Check sheet for the modelled part. Datum: model origin and axes. Units: mm. Face numbers are marked on the shaded views. A direction names the side the tool comes from. Give positions to 0.01 mm unless a question says otherwise; leave off trailing zeros. Write each loop counter-clockwise with the first axis right and the second up, starting at its lowest first coordinate (ties: lowest second). Pieces come first, ordered by that corner, then holes. Notation, with made-up numbers: M 51.25,37 L 74.25,37 A24 ccw 74.25,63 Z; hole C 77,86 d4. An arc over 180 degrees is marked long. Use CSV: the item, a comma, the result in double quotes. Start each with the question number.
1. Scan lines: line 1 (Y direction, x = 0, z = 17.65); line 2 (Y direction, x = 0, z = -13.1); line 3 (Z direction, x = -8, y = -4.5). Record each from-to range of solid material in increasing order.
2. Depth check by flat-ended pin: P1, Ø1.6, axis at x = -8, y = 0.5, coming from the +Z side; P2, Ø1.5, axis at x = -2, z = -9, coming from the +Y side; P3, Ø5, axis at y = 6.5, z = 13.5, coming from the -X side. Enter the tip coordinate at first touch or a pass-through.
3. Access from +Z, -Z, +X, -X, +Y, -Y to the whole of each face (thin tool, end or side, straight path). Record for the marked faces 1 and 2.
4. Cross-section at C-C, the plane z = -0.5. Enter the section's corners in (x, y), and give its area (3 significant figures).
5. Cross-section at B-B, the plane y = 8.5. Enter the section's corners in (x, z).
6. Cross-section at A-A, the plane x = 0. Enter the section's corners in (y, z).
7. Cross-section at D-D, the plane x = -8. Enter the section's corners in (y, z), and give its area (3 significant figures).
from build123d import *

# Parameters (mm, degrees)
SKETCH1_R                = 10.25
BOSS_EXTRUDE1_DEPTH      = 19
BOSS_EXTRUDE1_DEPTH_BACK = 19
SKETCH2_R                = 4
BOSS_EXTRUDE2_DEPTH      = 1.9
SKETCH3_R                = 4
BOSS_EXTRUDE3_DEPTH      = 1
SKETCH4_R                = 1
CUT_EXTRUDE1_DEPTH       = 3.5
FILLET1_R                = 0.5
SKETCH7_R                = 10.25
CUT_EXTRUDE3_DEPTH       = 5.5
CUT_EXTRUDE3_DEPTH_BACK  = 3.5
SKETCH9_R                = 1.5
CUT_EXTRUDE5_DEPTH       = 5


with BuildPart() as part:
    # Sketch1 → Boss-Extrude1 (new body, two sides)
    with BuildSketch(Plane.XY) as boss_extrude1_sk:
        Circle(SKETCH1_R)
    extrude(amount=BOSS_EXTRUDE1_DEPTH)
    extrude(boss_extrude1_sk.sketch, amount=-BOSS_EXTRUDE1_DEPTH_BACK)

    # Sketch2 → Boss-Extrude2 (add)
    with BuildSketch(Plane.XY.offset(19)):
        Circle(SKETCH2_R)
    extrude(amount=BOSS_EXTRUDE2_DEPTH)

    # Sketch3 → Boss-Extrude3 (add)
    with BuildSketch(Plane(origin=(0, 0, -19), x_dir=(-1, 0, 0), z_dir=(0, 0, -1))):
        Circle(SKETCH3_R)
    extrude(amount=BOSS_EXTRUDE3_DEPTH)

    # Sketch4 → Cut-Extrude1 (cut)
    with BuildSketch(Plane.XY.offset(19)):
        with Locations((0, 8)):
            Circle(SKETCH4_R)
        with Locations((8, 0)):
            Circle(SKETCH4_R)
        with Locations((0, -8)):
            Circle(SKETCH4_R)
        with Locations((-8, 0)):
            Circle(SKETCH4_R)
    cut_extrude1 = extrude(amount=-CUT_EXTRUDE1_DEPTH, mode=Mode.SUBTRACT)

    # Fillet1
    fillet1_edges = [part.edges().sort_by_distance(p)[0] for p in [
        (-4, 0, 20.9),
    ]]
    fillet(fillet1_edges, radius=FILLET1_R)

    # Mirror1: Cut-Extrude1 across plane
    add(cut_extrude1.mirror(Plane(origin=(0, 0, 0), x_dir=(1, 0, 0), z_dir=(0, 0, -1))), mode=Mode.SUBTRACT)

    # Sketch7 → Cut-Extrude3 (cut, two sides)
    with BuildSketch(Plane(origin=(0, 0, -19), x_dir=(-1, 0, 0), z_dir=(0, 0, -1))) as cut_extrude3_sk:
        Circle(SKETCH7_R)
    extrude(amount=CUT_EXTRUDE3_DEPTH, mode=Mode.SUBTRACT)
    extrude(cut_extrude3_sk.sketch, amount=-CUT_EXTRUDE3_DEPTH_BACK, mode=Mode.SUBTRACT)

    # Sketch9 → Cut-Extrude5 (cut)
    with BuildSketch(Plane(origin=(0, 0, -15.5), x_dir=(-1, 0, 0), z_dir=(0, 0, -1))):
        Circle(SKETCH9_R)
    extrude(amount=-CUT_EXTRUDE5_DEPTH, mode=Mode.SUBTRACT)


solid = part.part
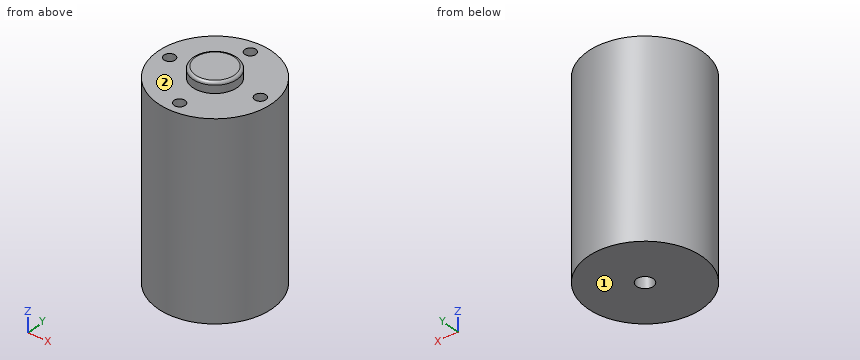
Worked answers:
1,line 1,"y = -10.25 to -9, -7 to 7, 9 to 10.25"
1,line 2,"y = -10.25 to -1.5, 1.5 to 10.25"
1,line 3,"z = -15.5 to 19"
2,P1,"stops at z = 19"
2,P2,"stops at y = 10.17"
2,P3,"stops at x = -9.44"
3,face 1,"-Z, +X, -X, +Y, -Y"
3,face 2,"+Z"
4,outline,"C 0,0 d20.5"
4,area,"330 mm^2"
5,outline,"M -5.73,-15.5 L 5.73,-15.5 L 5.73,19 L 0.87,19 L 0.87,15.5 L -0.87,15.5 L -0.87,19 L -5.73,19 Z"
6,outline,"M -10.25,-15.5 L -1.5,-15.5 L -1.5,-10.5 L 1.5,-10.5 L 1.5,-15.5 L 10.25,-15.5 L 10.25,19 L 9,19 L 9,15.5 L 7,15.5 L 7,19 L 4,19 L 4,20.4 A0.5 ccw 3.5,20.9 L -3.5,20.9 A0.5 ccw -4,20.4 L -4,19 L -7,19 L -7,15.5 L -9,15.5 L -9,19 L -10.25,19 Z"
7,outline,"M -6.41,-15.5 L 6.41,-15.5 L 6.41,19 L 1,19 L 1,15.5 L -1,15.5 L -1,19 L -6.41,19 Z"
7,area,"435 mm^2"
